Autodesk Inventor part; units mm, degrees
ref_plane "YZ Plane" through (0, 0, 0) normal (1, 0, 0) x (0, 1, 0)
ref_plane "XZ Plane" through (0, 0, 0) normal (0, 1, 0) x (-1, 0, 0)
ref_plane "XY Plane" through (0, 0, 0) normal (0, 0, 1) x (1, 0, 0)
sketch "Sketch1" plane through (0, 0, 0) normal (0, 1, 0) x (-1, 0, 0)
  line L0 (-100, 50) -> (100, 50)
  line L1 (100, 50) -> (100, -50)
  line L2 (100, -50) -> (-100, -50)
  line L3 (-100, -50) -> (-100, 50)
  line L4 (-100, 50) -> (100, -50) construction
  line L5 (100, 50) -> (-100, -50) construction
  point P0 (0, 0)
  dimension "d0" = 200
  dimension "d1" = 100
extrude "Extrusion1" add sketch "Sketch1" along normal blind 5
chamfer "Chamfer1" distance 15 angle 45 4 edges at (100, 2.5, -50) (100, 2.5, 50) (-100, 2.5, 50) (-100, 2.5, -50)
sketch "Sketch2" plane through (0, 5, 0) normal (0, 1, 0) x (1, 0, 0)
  line L0 (-85, -50) -> (85, -50)
  line L1 (85, 50) -> (85, -50)
  line L2 (85, 0) -> (0, 0)
  line L3 (85, 50) -> (-85, 50)
  line L4 (85, 0) -> (75, 0)
  line L5 (75, 0) -> (75, 50)
  line L6 (85, -50) -> (85, -45)
  line L7 (85, -45) -> (87.1749, -45)
  dimension "d7" = 10
  dimension "d15" = 5
hole "Hole2" at (85, 5, 45) direction (0, -1, 0) diameter 3.5 depth 12
pattern_linear "Rectangular Pattern1" count 10 spacing 10 along (0, 0, -1) of "Hole2"
mirror "Mirror1" about plane through (0, 0, 0) normal (1, 0, 0) of "Hole2", "Rectangular Pattern1"
properties part number "Chasis2"
Model file for the job. Use its own axes, mm. Coordinates: 2 decimals unless noted, no trailing zeros. Use CSV: the item, a comma, the result in double quotes. Start each with the question number.
1. Band-saw the part on A-A, the plane y = 3.2. Give the number of separate pieces and of enclosed holes in the cut face, then the cut area to 3 significant figures.
2. Two-plate mould, pull along X, no slides. Class faces 1 (the flat face through (93, 2, -42)), 2 (the flat face through (-93, 2, 42)), 3 (the flat face through (1, 5, 1)), 4 (the cylindrical face through (-83.29, 2.46, 14.62)): pulls with the +X half, pulls with the -X half, needs draft (parallel to the pull), parting line crosses it, or undercut.
3. Probe probe 1 along X at (y, z) = (3.95, -15); probe 2 along X at (y, z) = (2.95, 36.5); probe 3 along X at (y, z) = (2.2, 38). List the from-to ranges inside material, lowest first. Write a range as [from, to].
4. Flat gauge pin, fed straight in: pin 1 (3 mm diameter, centred on x = 85, z = 45, fed in from +Y). Where does the tip first touch, or does it go through?
Entries:
1,separate pieces,"1"
1,enclosed holes,"20"
1,area,"19,400 mm2"
2,face 1,"pulls with the +X half"
2,face 2,"pulls with the -X half"
2,face 3,"needs draft"
2,face 4,"undercut"
3,probe 1,"x = [-100, -86.75], [-83.25, 83.25], [86.75, 100]"
3,probe 2,"x = [-98.5, -85.9], [-84.1, 84.1], [85.9, 98.5]"
3,probe 3,"x = [-97, 97]"
4,pin 1,"passes through"
